CAD build for the part. Positions are in the model's coordinates, mm. Face numbers are marked on the shaded views. A direction names the side the tool comes from. Round coordinates to 2 decimals unless told otherwise and drop trailing zeros. Loops run counter-clockwise (first coordinate to the right, second up) from the corner with the lowest first, then second, coordinate; pieces in that order, holes last.
from build123d import *

# Parameters (mm, degrees)
SKETCH1_R           = 35
BOSS_EXTRUDE1_DEPTH = 23.5
SKETCH2_R           = 15
BOSS_EXTRUDE2_DEPTH = 25
CUT_EXTRUDE1_REACH  = 72.356
SKETCH3_R           = 10.5
CUT_EXTRUDE2_REACH  = 71.298
SKETCH4_R           = 2


with BuildPart() as part:
    # Sketch1 → Boss-Extrude1 (new, symmetric)
    with BuildSketch(Plane.XY):
        Circle(SKETCH1_R)
    extrude(amount=BOSS_EXTRUDE1_DEPTH, both=True)

    # Sketch2 → Boss-Extrude2 (add, symmetric)
    with BuildSketch(Plane.XY):
        Circle(SKETCH2_R)
    extrude(amount=BOSS_EXTRUDE2_DEPTH, both=True)

    # Sketch3 → Cut-Extrude1 (cut, up to next)
    with BuildSketch(Plane.XY.offset(25), mode=Mode.PRIVATE) as cut_extrude1_sk1:
        Circle(SKETCH3_R)
    cut_extrude1_tool1 = extrude(cut_extrude1_sk1.sketch, amount=-CUT_EXTRUDE1_REACH, mode=Mode.PRIVATE) & part.part
    add(cut_extrude1_tool1.solids().sort_by_distance((0, 0, 25))[0], mode=Mode.SUBTRACT)

    # Sketch4 → Cut-Extrude2 (cut, up to next)
    with BuildSketch(Plane.XY.offset(23.5), mode=Mode.PRIVATE) as cut_extrude2_sk1:
        with Locations((0, 25)):
            Circle(SKETCH4_R)
    cut_extrude2_tool1 = extrude(cut_extrude2_sk1.sketch, amount=-CUT_EXTRUDE2_REACH, mode=Mode.PRIVATE) & part.part
    # Sketch4 → Cut-Extrude2 (cut, up to next)
    with BuildSketch(Plane.XY.offset(23.5), mode=Mode.PRIVATE) as cut_extrude2_sk2:
        with Locations((21.650635095, -12.5)):
            Circle(SKETCH4_R)
    cut_extrude2_tool2 = extrude(cut_extrude2_sk2.sketch, amount=-CUT_EXTRUDE2_REACH, mode=Mode.PRIVATE) & part.part
    # Sketch4 → Cut-Extrude2 (cut, up to next)
    with BuildSketch(Plane.XY.offset(23.5), mode=Mode.PRIVATE) as cut_extrude2_sk3:
        with Locations((-21.650635095, -12.5)):
            Circle(SKETCH4_R)
    cut_extrude2_tool3 = extrude(cut_extrude2_sk3.sketch, amount=-CUT_EXTRUDE2_REACH, mode=Mode.PRIVATE) & part.part
    add(cut_extrude2_tool1.solids().sort_by_distance((0, 25, 23.5))[0], mode=Mode.SUBTRACT)
    add(cut_extrude2_tool2.solids().sort_by_distance((21.650635, -12.5, 23.5))[0], mode=Mode.SUBTRACT)
    add(cut_extrude2_tool3.solids().sort_by_distance((-21.650635, -12.5, 23.5))[0], mode=Mode.SUBTRACT)


solid = part.part
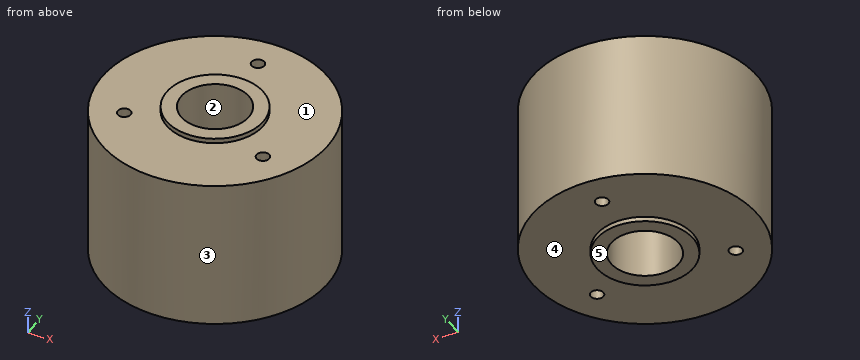
Item 1: Flat gauge pins, fed straight in: P1, Ø8, axis at y = 17.5, z = -9, coming from the -X side; P2, Ø3, axis at x = -5.5, z = 15, coming from the -Y side; P3, Ø1, axis at y = -10.5, z = 1.5, coming from the +X side. Where does each tip first touch, or does it go through?
Verdict:
P1: stops at x = -32.29
P2: stops at y = -34.77
P3: stops at x = 33.54
Item 2: 3-axis set-ups, long thin cutter, end or side, ignore diameter. For the marked faces 4 and 5: which of +Z, -Z, +X, -X, +Y, -Y reach the whole face in a straight line?
Verdict:
face 4: -Z
face 5: -Z, +X, -X, +Y, -Y
Item 3: Cut at D-D (y = -12.5). List the corners of the cut face in (x, z), plus the area to 3 significant figures.
Verdict:
outline: (-32.69, -23.5) - (-23.65, -23.5) - (-23.65, 23.5) - (-32.69, 23.5) - close; (-19.65, -23.5) - (-8.29, -23.5) - (-8.29, -25) - (8.29, -25) - (8.29, -23.5) - (19.65, -23.5) - (19.65, 23.5) - (8.29, 23.5) - (8.29, 25) - (-8.29, 25) - (-8.29, 23.5) - (-19.65, 23.5) - close; (23.65, -23.5) - (32.69, -23.5) - (32.69, 23.5) - (23.65, 23.5) - close
area: 2,750 mm2
Item 4: Cut at C-C (z = 18.5). List the corners of the cut face in (x, y), plus the area to 3 significant figures.
Verdict:
outline: circle Ø70 at (0, 0); hole circle Ø4 at (-21.65, -12.5); hole circle Ø21 at (0, 0); hole circle Ø4 at (0, 25); hole circle Ø4 at (21.65, -12.5)
area: 3,460 mm2
Item 5: Cut at B-B (x = 0). List the corners of the cut face in (y, z), plus the area to 3 significant figures.
Verdict:
outline: (-35, -23.5) - (-15, -23.5) - (-15, -25) - (-10.5, -25) - (-10.5, 25) - (-15, 25) - (-15, 23.5) - (-35, 23.5) - close; (10.5, -25) - (15, -25) - (15, -23.5) - (23, -23.5) - (23, 23.5) - (15, 23.5) - (15, 25) - (10.5, 25) - close; (27, -23.5) - (35, -23.5) - (35, 23.5) - (27, 23.5) - close
area: 2,140 mm2
Item 6: Wall check: L1, parallel to Y at x = 0, z = -13; L2, parallel to Z at x = 22, y = 21; L3, parallel to X at y = -5.5, z = -7. Give the ranges that are in metal, low to high.
Verdict:
L1: y = -35 to -10.5, 10.5 to 23, 27 to 35
L2: z = -23.5 to 23.5
L3: x = -34.57 to -8.94, 8.94 to 34.57
Item 7: Mould opens along Y. For the marked faces 1, 2 and 3 say: released by +Y, released by -Y, zero draft, split by the parting line, or undercut.
Verdict:
face 1: zero draft
face 2: undercut
face 3: split by the parting line
Item 8: Cut at A-A (y = 0). List the corners of the cut face in (x, z), plus the area to 3 significant figures.
Verdict:
outline: (-35, -23.5) - (-15, -23.5) - (-15, -25) - (-10.5, -25) - (-10.5, 25) - (-15, 25) - (-15, 23.5) - (-35, 23.5) - close; (10.5, -25) - (15, -25) - (15, -23.5) - (35, -23.5) - (35, 23.5) - (15, 23.5) - (15, 25) - (10.5, 25) - close
area: 2,330 mm2
